from build123d import *

# Parameters (mm, degrees)
SKETCH1_R           = 0.89
SKETCH1_R_2         = 2
SKETCH1_W           = 3.27
SKETCH1_H           = 0.75
BOSS_EXTRUDE1_DEPTH = 2.5
SKETCH2_R           = 0.89
BOSS_EXTRUDE2_DEPTH = 6
FILLET1_R           = 0.5


with BuildPart() as part:
    # Sketch1 → Boss-Extrude1 (new body)
    # profile 1 of 7: a face of its own
    with BuildSketch(Plane(origin=(0, 0, 0), x_dir=(1, 0, 0), z_dir=(0, 1, 0))):
        Polygon((0, 17.78), (0, 0), (3.27, 0), (3.27, 3.2), (39.91, 3.2), (39.91, 0), (43.18, 0), (43.18, 17.78), (39.91, 17.78), (39.91, 14.58), (3.27, 14.58), (3.27, 17.78), align=None)
        with Locations(Location((1.27, 1.27, 0), (0, 0, 270))):
            Circle(SKETCH1_R, mode=Mode.SUBTRACT)
        with Locations(Location((41.91, 1.27, 0), (0, 0, 270))):
            Circle(SKETCH1_R, mode=Mode.SUBTRACT)
        with Locations(Location((1.27, 16.51, 0), (0, 0, 270))):
            Circle(SKETCH1_R, mode=Mode.SUBTRACT)
        with Locations(Location((41.91, 16.51, 0), (0, 0, 270))):
            Circle(SKETCH1_R, mode=Mode.SUBTRACT)
    # profile 2 of 7: a face of its own
    with BuildSketch(Plane(origin=(0, 0, 0), x_dir=(1, 0, 0), z_dir=(0, 1, 0))):
        Polygon((0, -0.75), (0, 0), (0, 17.78), (0, 18.53), (0, 20.01), (-9, 20.01), (-9, -2.23), (0, -2.23), align=None)
        with Locations(Location((-4.5, 1.27, 0), (0, 0, 270))):
            Circle(SKETCH1_R_2, mode=Mode.SUBTRACT)
        with Locations(Location((-4.5, 16.51, 0), (0, 0, 270))):
            Circle(SKETCH1_R_2, mode=Mode.SUBTRACT)
    # profile 3 of 7: a face of its own
    with BuildSketch(Plane(origin=(0, 0, 0), x_dir=(1, 0, 0), z_dir=(0, 1, 0))):
        Polygon((43.18, 17.78), (43.18, 0), (43.18, -0.75), (43.18, -2.23), (52.18, -2.23), (52.18, 20.01), (43.18, 20.01), (43.18, 18.53), align=None)
        with Locations(Location((47.68, 1.27, 0), (0, 0, 270))):
            Circle(SKETCH1_R_2, mode=Mode.SUBTRACT)
        with Locations(Location((47.68, 16.51, 0), (0, 0, 270))):
            Circle(SKETCH1_R_2, mode=Mode.SUBTRACT)
    # profile 4 of 7: a face of its own
    with BuildSketch(Plane(origin=(0, 0, 0), x_dir=(1, 0, 0), z_dir=(0, 1, 0))):
        with Locations((41.545, -0.375)):
            Rectangle(SKETCH1_W, SKETCH1_H)
    # profile 5 of 7: a face of its own
    with BuildSketch(Plane(origin=(0, 0, 0), x_dir=(1, 0, 0), z_dir=(0, 1, 0))):
        with Locations((41.545, 18.155)):
            Rectangle(SKETCH1_W, SKETCH1_H)
    # profile 6 of 7: a face of its own
    with BuildSketch(Plane(origin=(0, 0, 0), x_dir=(1, 0, 0), z_dir=(0, 1, 0))):
        with Locations((1.635, 18.155)):
            Rectangle(SKETCH1_W, SKETCH1_H)
    # profile 7 of 7: a face of its own
    with BuildSketch(Plane(origin=(0, 0, 0), x_dir=(1, 0, 0), z_dir=(0, 1, 0))):
        with Locations((1.635, -0.375)):
            Rectangle(SKETCH1_W, SKETCH1_H)
    extrude(amount=BOSS_EXTRUDE1_DEPTH)

    # Sketch2 → Boss-Extrude2 (add)
    with BuildSketch(Plane.XZ):
        with Locations(Location((1.27, -16.51, 0), (0, 0, 270))):
            Circle(SKETCH2_R)
        with Locations(Location((1.27, -1.27, 0), (0, 0, 270))):
            Circle(SKETCH2_R)
        with Locations(Location((41.91, -16.51, 0), (0, 0, 270))):
            Circle(SKETCH2_R)
        with Locations(Location((41.91, -1.27, 0), (0, 0, 270))):
            Circle(SKETCH2_R)
    extrude(amount=-BOSS_EXTRUDE2_DEPTH)

    # Fillet1
    fillet1_edges = [part.edges().sort_by_distance(p)[0] for p in [
        (41.91, 2.5, -0.38),
        (41.91, 2.5, -15.62),
        (1.27, 2.5, -0.38),
        (1.27, 2.5, -15.62),
    ]]
    fillet(fillet1_edges, radius=FILLET1_R)


solid = part.part
Work out the finished part from the listing and answer in its coordinate system (mm). A direction names the side the tool comes from. Round coordinates to 2 decimals unless told otherwise and drop trailing zeros. Write each loop counter-clockwise with the first axis right and the second up, starting at its lowest first coordinate (ties: lowest second). Pieces come first, ordered by that corner, then holes. Notation, with made-up numbers: (-29.5, 14) - (-19.5, 14) arc R19 cw to (-19.5, 18) - close; hole circle Ø1 at (10.5, 82.25). An arc over 180 degrees is marked (long way). Answer in a Markdown table with one row per item. Add a question column.
1. Find the intervals of material crossed by line 1 along X through (y, z) = (1.85, -16.51); line 2 along X through (y, z) = (0.6, 0.5); line 3 along Y through (x, z) = (36, -6.75), in increasing order. Write a range as from..to.
2. A cutting plane is placed at C-C, the plane x = 47.68. Determine the outline of the cut face in (y, z).
3. For faces 1 (the flat face through (2, 1, 0.75)), 2 (the flat face through (48, 1, 2.23)), 3 (the flat face through (2, 1, -18.53)), 4 (the cylindrical face through (1.54, 4.48, -17.36)), determine the directions among +Z, -Z, +X, -X, +Y, -Y from which every point of the face is accessible in a straight line to the end or side of a thin tool.
4. A cutting plane is placed at D-D, the plane x = 21.5. Determine the outline of the cut face in (y, z), and give its area (4 significant figures).
5. The mould has two halves that part along Z. Classify faces 5 (the cylindrical face through (0.929, 4.479, -2.092)), 6 (the flat face through (0, 1, -19)), 7 (the flat face through (-4, 1, -20.01)): +Z half, -Z half, draft (parallel to the pull), parting line (faces both ways), or undercut.
6. Given pin 1 (6 mm diameter, centred on x = 5, z = -17.5, fed in from -Y); pin 2 (3 mm diameter, centred on x = 41.5, y = 2, fed in from +Z); pin 3 (0.8 mm diameter, centred on x = 20.5, y = 1, fed in from -Z); pin 4 (1.5 mm diameter, centred on x = 0, z = -4.5, fed in from +Y), each flat-ended and moving along its own axis, determine where each tip first touches the part or whether it passes through.
7. A cutting plane is placed at A-A, the plane z = -1.27. Determine the outline of the cut face in (x, y), and give its area (3 significant figures).
8. A cutting plane is placed at B-B, the plane y = 1.8. Determine the outline of the cut face in (x, z), and give its area (3 significant figures).
Worked out:
| question | item | result |
|---|---|---|
| 1 | line 1 | -9..-6.5, -2.5..3.27, 39.91..45.68, 49.68..52.18 |
| 1 | line 2 | -9..-5.43, -3.57..3.27, 39.91..46.75, 48.61..52.18 |
| 1 | line 3 | 0..2.5 |
| 2 | outline | (0, -20.01) - (2.5, -20.01) - (2.5, -18.51) - (0, -18.51) - close; (0, -14.51) - (2.5, -14.51) - (2.5, -3.27) - (0, -3.27) - close; (0, 0.73) - (2.5, 0.73) - (2.5, 2.23) - (0, 2.23) - close |
| 3 | face 1 | +Z, +Y, -Y |
| 3 | face 2 | +Z, +X, -X, +Y, -Y |
| 3 | face 3 | -Z, +Y, -Y |
| 3 | face 4 | +Y |
| 4 | outline | (0, -14.58) - (2.5, -14.58) - (2.5, -3.2) - (0, -3.2) - close |
| 4 | area | 28.45 mm^2 |
| 5 | face 5 | undercut |
| 5 | face 6 | draft |
| 5 | face 7 | -Z half |
| 6 | pin 1 | y = 0 |
| 6 | pin 2 | z = 0.75 |
| 6 | pin 3 | z = -14.58 |
| 6 | pin 4 | y = 2.5 |
| 7 | outline | (-9, 0) - (-6.5, 0) - (-6.5, 2.5) - (-9, 2.5) - close; (-2.5, 0) - (3.27, 0) - (3.27, 2.5) - (2.66, 2.5) arc R0.5 cw to (2.16, 3) - (2.16, 6) - (0.38, 6) - (0.38, 3) arc R0.5 cw to (-0.12, 2.5) - (-2.5, 2.5) - close; (39.91, 0) - (45.68, 0) - (45.68, 2.5) - (43.3, 2.5) arc R0.5 cw to (42.8, 3) - (42.8, 6) - (41.02, 6) - (41.02, 3) arc R0.5 cw to (40.52, 2.5) - (39.91, 2.5) - close; (49.68, 0) - (52.18, 0) - (52.18, 2.5) - (49.68, 2.5) - close |
| 7 | area | 54.0 mm^2 |
| 8 | outline | (-9, -20.01) - (0, -20.01) - (0, -18.53) - (3.27, -18.53) - (3.27, -14.58) - (39.91, -14.58) - (39.91, -18.53) - (43.18, -18.53) - (43.18, -20.01) - (52.18, -20.01) - (52.18, 2.23) - (43.18, 2.23) - (43.18, 0.75) - (39.91, 0.75) - (39.91, -3.2) - (3.27, -3.2) - (3.27, 0.75) - (0, 0.75) - (0, 2.23) - (-9, 2.23) - close; hole circle Ø4 at (-4.5, -16.51); hole circle Ø4 at (-4.5, -1.27); hole circle Ø4 at (47.68, -16.51); hole circle Ø4 at (47.68, -1.27) |
| 8 | area | 893 mm^2 |
